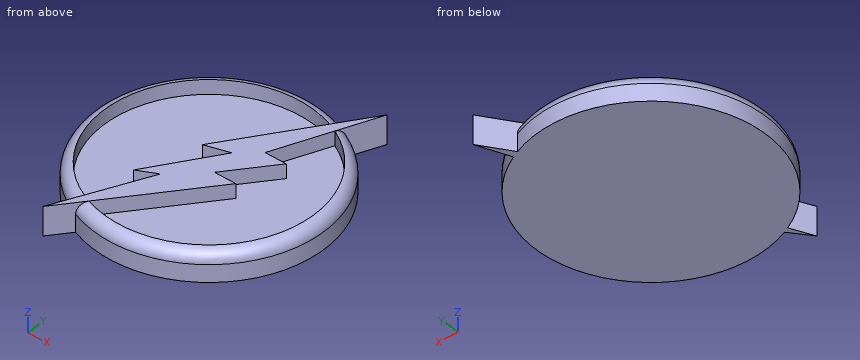
from build123d import *

# Parameters (mm, degrees)
F0_R     = 46.303997109
F1_DEPTH = 6.35
F0_R_2   = 50.7773250867
F2_DEPTH = 12.7
F5_DEPTH = 6.35
F6_DEPTH = 12.7


# Not quite as in the source:
# - a fillet or chamfer that OpenCascade refuses, or shapes differently, is made with other operations: its cross-section is extruded or revolved along the edge and cut away or added


with BuildPart() as f1:
    # F0 (on Top) → F1 (new body)
    with BuildSketch(Plane.XY):
        Circle(F0_R)
    extrude(amount=F1_DEPTH)

    # F0 (on Top) → F2 (join)
    with BuildSketch(Plane.XY):
        Circle(F0_R_2)
        Circle(F0_R, mode=Mode.SUBTRACT)
    extrude(amount=F2_DEPTH)

    # F3: fillet of radius 5.08 on 1 edges, made by hand

    # F3_s1 → F3_t2 (revolve, cut)
    with BuildSketch(Plane.XZ):
        with BuildLine():
            ThreePointArc((50.7773250867, 7.6563555778), (49.4978706971, 11.0271497073), (46.303997109, 12.7))
            Line((46.303997109, 12.7), (46.3161305494, 12.8008728884))
            ThreePointArc((46.3161305494, 12.8008728884), (48.5406610978, 12.8016), (50.7773250867, 12.8016))
            Line((50.7773250867, 12.8016), (50.8789250867, 12.7))
            Line((50.8789250867, 12.7), (50.8789250867, 7.6563555778))
            Line((50.8789250867, 7.6563555778), (50.7773250867, 7.6563555778))
        make_face()
    revolve(axis=Axis((0, 0, 12.7), (0, 0, 1)), mode=Mode.SUBTRACT)

    # F4 (on face) → F5 (join)
    with BuildSketch(Plane.XY.offset(6.35)):
        Polygon((-8.1779062748, -15.8028278183), (-26.3735784938, -55.8334334653), (14.7386826575, -3.0078946147), (5.1134219393, -3.0078946147), (20.4086864271, 16.6451374931), (10.8284205198, 16.6451374931), (28.2742083073, 59.8571076989), (-8.1779062748, 5.9409798123), (2.4016224779, 9.0941041708), (-16.5434218943, -20.15289478), align=None)
    extrude(amount=F5_DEPTH)

    # F6 (add): a face of the model
    f6_faces = [f1.faces().sort_by_distance(p)[0] for p in [
        (2.0188421937, 0.3767409736, 12.7),
    ]]
    extrude(f6_faces, amount=-F6_DEPTH)


solid = f1.part
CAD build for the part. Positions are in the model's coordinates, mm. Round coordinates to 2 decimals unless told otherwise and drop trailing zeros. Order: outer loops, then holes, each group sorted by start corner. A loop starts at its lowest first (then second) coordinate and runs counter-clockwise, first axis right, second up. Notation, with made-up numbers: (32, -9.75) -> (72, -9.75) arc R28 cw to (72, 20.25) -> close; hole circle Ø2 at (-11, -9). An arc over 180 degrees is marked (long way). Write each question's results on one line, items separated by ' | '.
1. Wall check: line 1 along Y through (x, z) = (-11, 7); line 2 along Y through (x, z) = (0, 7.5); line 3 along Z through (x, y) = (24, 9). Give the ranges that are in metal, low to high. Write a range as [from, to].
Findings below:
line 1: y = [-49.57, -44.98], [-36.08, -22.01], [-17.27, -11.6], [44.98, 49.57] | line 2: y = [-50.78, -46.3], [-21.95, 5.39], [8.38, 18.04], [46.3, 50.78] | line 3: z = [0, 6.35]
2. Cut at C-C (x = 0). Give the cut face in (y, z), plus the area to 3 significant figures.
Findings below:
outline: (-50.78, 0) -> (50.78, 0) -> (50.78, 7.66) arc R5.08 ccw to (46.3, 12.7) -> (46.3, 6.35) -> (18.04, 6.35) -> (18.04, 12.7) -> (8.38, 12.7) -> (8.38, 6.35) -> (5.39, 6.35) -> (5.39, 12.7) -> (-21.95, 12.7) -> (-21.95, 6.35) -> (-46.3, 6.35) -> (-46.3, 12.7) arc R5.08 ccw to (-50.78, 7.66) -> close | area: 926 mm²
3. Flat gauge pins, fed straight in: P1, Ø7, axis at x = 13.5, z = 10, coming from the +Y side; P2, Ø1.5, axis at y = 1.5, z = 6.5, coming from the -X side; P3, Ø1.9, axis at x = 10.5, z = 8.5, coming from the +Y side. Where does each tip first touch, or does it go through?
Findings below:
P1: stops at y = 49.65 | P2: stops at x = -50.77 | P3: stops at y = 49.83
4. Cut at A-A (y = 0). Give the cut face in (x, z).
Findings below:
outline: (-50.78, 0) -> (50.78, 0) -> (50.78, 7.66) arc R5.08 ccw to (46.3, 12.7) -> (46.3, 6.35) -> (7.45, 6.35) -> (7.45, 12.7) -> (-3.49, 12.7) -> (-3.49, 6.35) -> (-46.3, 6.35) -> (-46.3, 12.7) arc R5.08 ccw to (-50.78, 7.66) -> close
